```python
from build123d import *

# Parameters (mm, degrees)
ESTRUSIONE_ESTRUSIONE1_DEPTH  = 10
SCHIZZO10_W                   = 10
SCHIZZO10_H                   = 10
ESTRUSIONE_ESTRUSIONE4_DEPTH  = 140
SCHIZZO11_W                   = 10
SCHIZZO11_H                   = 10
ESTRUSIONE_ESTRUSIONE5_DEPTH  = 140
SCHIZZO12_W                   = 10
SCHIZZO12_H                   = 10
ESTRUSIONE_ESTRUSIONE6_DEPTH  = 100
SCHIZZO13_W                   = 10
SCHIZZO13_H                   = 10
ESTRUSIONE_ESTRUSIONE7_DEPTH  = 140
SCHIZZO16_W                   = 10
SCHIZZO16_H                   = 10
ESTRUSIONE_ESTRUSIONE8_DEPTH  = 140
SCHIZZO17_W                   = 10
SCHIZZO17_H                   = 10
ESTRUSIONE_ESTRUSIONE9_DEPTH  = 140
SCHIZZO19_W                   = 10
SCHIZZO19_H                   = 10
ESTRUSIONE_ESTRUSIONE10_DEPTH = 100
SCHIZZO20_W                   = 10
SCHIZZO20_H                   = 10
ESTRUSIONE_ESTRUSIONE11_DEPTH = 140
SCHIZZO21_W                   = 10
SCHIZZO21_H                   = 10
ESTRUSIONE_ESTRUSIONE12_DEPTH = 140
SCHIZZO22_W                   = 10
SCHIZZO22_H                   = 10
ESTRUSIONE_ESTRUSIONE13_DEPTH = 110
SCHIZZO23_W                   = 10
SCHIZZO23_H                   = 10
ESTRUSIONE_ESTRUSIONE14_DEPTH = 140
SCHIZZO24_W                   = 10
SCHIZZO24_H                   = 10
ESTRUSIONE_ESTRUSIONE15_DEPTH = 110
SCHIZZO25_W                   = 10
SCHIZZO25_H                   = 10
ESTRUSIONE_ESTRUSIONE16_DEPTH = 140
SCHIZZO26_W                   = 10
SCHIZZO26_H                   = 10
ESTRUSIONE_ESTRUSIONE17_DEPTH = 140


with BuildPart() as part:
    # Schizzo1 → Estrusione-Estrusione1 (new body)
    with BuildSketch(Plane.XY):
        Polygon((45, -75), (-75, -75), (-75, 75), (75, 75), (75, -45), (65, -45), (65, 65), (-65, 65), (-65, -65), (45, -65), align=None)
    extrude(amount=ESTRUSIONE_ESTRUSIONE1_DEPTH)

    # Schizzo10 → Estrusione-Estrusione4 (add)
    with BuildSketch(Plane.XY.offset(10)):
        with Locations((40, -70)):
            Rectangle(SCHIZZO10_W, SCHIZZO10_H)
    extrude(amount=ESTRUSIONE_ESTRUSIONE4_DEPTH)

    # Schizzo11 → Estrusione-Estrusione5 (add)
    with BuildSketch(Plane.ZY.offset(-35)):
        with Locations((145, -70)):
            Rectangle(SCHIZZO11_W, SCHIZZO11_H)
    extrude(amount=ESTRUSIONE_ESTRUSIONE5_DEPTH)

    # Schizzo12 → Estrusione-Estrusione6 (add)
    with BuildSketch(Plane(origin=(0, 0, 140), x_dir=(-1, 0, 0), z_dir=(0, 0, -1))):
        with Locations((100, -70)):
            Rectangle(SCHIZZO12_W, SCHIZZO12_H)
    extrude(amount=ESTRUSIONE_ESTRUSIONE6_DEPTH)

    # Schizzo13 → Estrusione-Estrusione7 (add)
    with BuildSketch(Plane(origin=(0, -65, 0), x_dir=(1, 0, 0), z_dir=(0, 1, 0))):
        with Locations((-100, -45)):
            Rectangle(SCHIZZO13_W, SCHIZZO13_H)
    extrude(amount=ESTRUSIONE_ESTRUSIONE7_DEPTH)

    # Schizzo16 → Estrusione-Estrusione8 (add)
    with BuildSketch(Plane.XY.offset(10)):
        with Locations((70, -40)):
            Rectangle(SCHIZZO16_W, SCHIZZO16_H)
    extrude(amount=ESTRUSIONE_ESTRUSIONE8_DEPTH)

    # Schizzo17 → Estrusione-Estrusione9 (add)
    with BuildSketch(Plane(origin=(0, -35, 0), x_dir=(1, 0, 0), z_dir=(0, 1, 0))):
        with Locations((70, -145)):
            Rectangle(SCHIZZO17_W, SCHIZZO17_H)
    extrude(amount=ESTRUSIONE_ESTRUSIONE9_DEPTH)

    # Schizzo19 → Estrusione-Estrusione10 (add)
    with BuildSketch(Plane(origin=(0, 0, 140), x_dir=(-1, 0, 0), z_dir=(0, 0, -1))):
        with Locations((-70, 100)):
            Rectangle(SCHIZZO19_W, SCHIZZO19_H)
    extrude(amount=ESTRUSIONE_ESTRUSIONE10_DEPTH)

    # Schizzo20 → Estrusione-Estrusione11 (add)
    with BuildSketch(Plane.ZY.offset(-65)):
        with Locations((45, 100)):
            Rectangle(SCHIZZO20_W, SCHIZZO20_H)
    extrude(amount=ESTRUSIONE_ESTRUSIONE11_DEPTH)

    # Schizzo21 → Estrusione-Estrusione12 (add)
    with BuildSketch(Plane.XY.offset(50)):
        with Locations((-70, 100)):
            Rectangle(SCHIZZO21_W, SCHIZZO21_H)
    extrude(amount=ESTRUSIONE_ESTRUSIONE12_DEPTH)

    # Schizzo22 → Estrusione-Estrusione13 (add)
    with BuildSketch(Plane(origin=(-65, 0, 0), x_dir=(0, 0, -1), z_dir=(1, 0, 0))):
        with Locations((-185, 100)):
            Rectangle(SCHIZZO22_W, SCHIZZO22_H)
    extrude(amount=ESTRUSIONE_ESTRUSIONE13_DEPTH)

    # Schizzo23 → Estrusione-Estrusione14 (add)
    with BuildSketch(Plane.XY.offset(50)):
        with Locations((-100, 70)):
            Rectangle(SCHIZZO23_W, SCHIZZO23_H)
    extrude(amount=ESTRUSIONE_ESTRUSIONE14_DEPTH)

    # Schizzo24 → Estrusione-Estrusione15 (add)
    with BuildSketch(Plane.XZ.offset(-65)):
        with Locations((-100, 185)):
            Rectangle(SCHIZZO24_W, SCHIZZO24_H)
    extrude(amount=ESTRUSIONE_ESTRUSIONE15_DEPTH)

    # Schizzo25 → Estrusione-Estrusione16 (add)
    with BuildSketch(Plane(origin=(-95, 0, 0), x_dir=(0, 0, -1), z_dir=(1, 0, 0))):
        with Locations((-185, -40)):
            Rectangle(SCHIZZO25_W, SCHIZZO25_H)
    extrude(amount=ESTRUSIONE_ESTRUSIONE16_DEPTH)

    # Schizzo26 → Estrusione-Estrusione17 (add)
    with BuildSketch(Plane.XZ.offset(-95)):
        with Locations((40, 185)):
            Rectangle(SCHIZZO26_W, SCHIZZO26_H)
    extrude(amount=ESTRUSIONE_ESTRUSIONE17_DEPTH)


solid = part.part
```
Build history of the part. All positions in model axes, mm. A direction names the side the tool comes from. Coordinates: 2 decimals unless noted, no trailing zeros. Order: outer loops, then holes, each group sorted by start corner. A loop starts at its lowest first (then second) coordinate and runs counter-clockwise, first axis right, second up.
Item 1: Saw through at C-C on x = 57. List the corners of the cut face in (y, z), then the cut area to 3 significant figures.
Filled in:
outline: (65, 0) - (75, 0) - (75, 10) - (65, 10) - close; (95, 40) - (105, 40) - (105, 50) - (95, 50) - close
area: 200 mm2
Item 2: Drop flat-ended pins along their axis: pin 1 Ø5 at (y, z) = (-71, 56.5) entering from +X; pin 2 Ø11 at (x, z) = (72, 60.5) entering from -Y; pin 3 Ø8 at (y, z) = (101, 133.5) entering from -X. Give the stop position or say it passes through.
Filled in:
pin 1: stops at x = 45
pin 2: stops at y = -45
pin 3: stops at x = -75
Item 3: Saw through at B-B on z = 146.5. List the corners of the cut face in (x, y), then the cut area to 3 significant figures.
Filled in:
outline: (-105, -75) - (45, -75) - (45, -65) - (-105, -65) - close; (-105, 65) - (-95, 65) - (-95, 75) - (-105, 75) - close; (-75, 95) - (-65, 95) - (-65, 105) - (-75, 105) - close; (65, -45) - (75, -45) - (75, 105) - (65, 105) - close
area: 3,200 mm2
Item 4: Saw through at A-A on y = 35.5. List the corners of the cut face in (x, z).
Filled in:
outline: (-105, 40) - (-95, 40) - (-95, 50) - (-105, 50) - close; (-105, 180) - (-95, 180) - (-95, 190) - (-105, 190) - close; (-75, 0) - (-65, 0) - (-65, 10) - (-75, 10) - close; (35, 180) - (45, 180) - (45, 190) - (35, 190) - close; (65, 0) - (75, 0) - (75, 10) - (65, 10) - close; (65, 140) - (75, 140) - (75, 150) - (65, 150) - close
Item 5: Tool access for faces 1 (the flat face through (-75, 100, 114)), 2 (the flat face through (65, 19, 142)), 3 (the flat face through (36, 19, 180)), 4 (the flat face through (70, -45, 74)): list every direction of +Z, -Z, +X, -X, +Y, -Y with a clear straight run to the whole face (end or side of a thin tool).
Filled in:
face 1: +Z, -Z, -X, +Y
face 2: +Z, -Y
face 3: +X, -Y
face 4: +Z, -Z, +X, -Y
Item 6: Drill centre lines: L1, parallel to Z at x = 1, y = -36; L2, parallel to Y at x = 42, z = 117; L3, parallel to Z at x = 51, y = 69.5. Where is each one in solid material? Low to high.
Filled in:
L1: z = 180 to 190
L2: y = -75 to -65
L3: z = 0 to 10
Item 7: Mould opens along Z. For faces 5 (the flat face through (-65, 1, 5)), 6 (the flat face through (-100, -1, 50)), 7 (the flat face through (70, 29, 150)) say: released by +Z, released by -Z, zero draft, split by the parting line, or undercut.
Filled in:
face 5: zero draft
face 6: undercut
face 7: released by +Z
Item 8: Saw through at D-D on y = -60. List the corners of the cut face in (x, z).
Filled in:
outline: (-105, 40) - (-95, 40) - (-95, 50) - (-105, 50) - close; (-75, 0) - (-65, 0) - (-65, 10) - (-75, 10) - close
